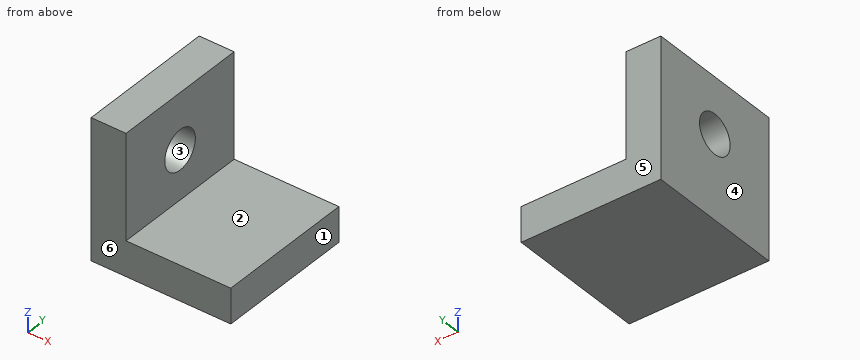
Autodesk Fusion 360 part; units mm, degrees
sketch "Sketch1" plane through (0, 0, 0) normal (0, 0, 1) x (1, 0, 0)
  line L0 (0, 0) -> (25.4, 0)
  line L1 (25.4, 0) -> (25.4, 25.4)
  line L2 (25.4, 25.4) -> (0, 25.4)
  line L3 (0, 25.4) -> (0, 0)
  line L4 (0, 25.4) -> (6.35, 25.4)
  line L5 (6.35, 25.4) -> (6.35, 0)
  line L6 (6.35, 0) -> (0, 0)
  line L7 (0, 0) -> (0, 25.4)
  dimension "d1" = 25.4
  dimension "d2" = 25.4
  dimension "d3" = 6.35
extrude "Extrude1" add sketch "Sketch1" along normal blind 6.35 contours L0 L1 L2 L5
extrude "Extrude2" add sketch "Sketch1" along normal blind 25.4 contours L0 L2 L3 L4 L5 L6 L7
sketch "Sketch2" plane through (6.35, 0, 0) normal (1, 0, 0) x (0, 1, 0)
  line L0 (0, 6.35) -> (25.4, 6.35)
  line L1 (25.4, 6.35) -> (25.4, 25.4)
  line L2 (25.4, 25.4) -> (0, 25.4)
  line L3 (0, 25.4) -> (0, 6.35)
  circle A0 centre (12.7, 15.24) radius 3.5921
extrude "Extrude3" cut sketch "Sketch2" against normal blind 38.1 contours A0
For this review, take the finished solid that the model builds, in its own axes (mm). Face numbers are marked on the shaded views. A direction names the side the tool comes from. Give positions to 0.01 mm unless a question says otherwise; leave off trailing zeros. Loops run counter-clockwise (first coordinate to the right, second up) from the corner with the lowest first, then second, coordinate; pieces in that order, holes last.
Item 1: Take a section at C-C, the plane y = 10. State the section outline as (x, z) points, and give its area (3 significant figures).
Item 2: Insertion check: pin 1 (6 mm diameter, centred on y = 14, z = 22, fed in from +X); pin 2 (5.5 mm diameter, centred on x = 18.5, y = 7.5, fed in from +Z). Each pin has a flat end and moves straight along its axis. Give the tip position at first contact, or say it passes through.
Item 3: Take a section at B-B, the plane z = 15.24. State the section outline as (x, y) points, and give its area (3 significant figures).
Item 4: For line 1 along Z through (x, y) = (2.75, 12.7); line 2 along Z through (x, y) = (20.75, 13.5), list the stretches that pass through material, from the lowest coordinate up.
Item 5: Take a section at A-A, the plane y = 12.7. State the section outline as (x, z) points, and give its area (3 significant figures).
Item 6: Take a section at D-D, the plane z = 10.75. State the section outline as (x, y) points, and give its area (3 significant figures).
Item 7: Tool access review of the marked faces 1 and 2: name each direction out of +Z, -Z, +X, -X, +Y, -Y from which nothing blocks a thin tool from reaching the whole face with its end or side.
Item 8: Draft analysis for pull direction Y (two halves, no side actions). For the marked faces 3, 4, 5 and 6, state which applies: +Y half, -Y half, draft (parallel to the pull), parting line (faces both ways), or undercut.
Calculated:
1. outline: (0, 0) - (25.4, 0) - (25.4, 6.35) - (6.35, 6.35) - (6.35, 12.87) - (0, 12.87) - close; (0, 17.61) - (6.35, 17.61) - (6.35, 25.4) - (0, 25.4) - close
1. area: 252 mm2
2. pin 1: stops at x = 6.35
2. pin 2: stops at z = 6.35
3. outline: (0, 0) - (6.35, 0) - (6.35, 9.11) - (0, 9.11) - close; (0, 16.29) - (6.35, 16.29) - (6.35, 25.4) - (0, 25.4) - close
3. area: 116 mm2
4. line 1: z = 0 to 11.65, 18.83 to 25.4
4. line 2: z = 0 to 6.35
5. outline: (0, 0) - (25.4, 0) - (25.4, 6.35) - (6.35, 6.35) - (6.35, 11.65) - (0, 11.65) - close; (0, 18.83) - (6.35, 18.83) - (6.35, 25.4) - (0, 25.4) - close
5. area: 237 mm2
6. outline: (0, 0) - (6.35, 0) - (6.35, 25.4) - (0, 25.4) - close
6. area: 161 mm2
7. face 1: +Z, -Z, +X, +Y, -Y
7. face 2: +Z, +X, +Y, -Y
8. face 3: undercut
8. face 4: draft
8. face 5: +Y half
8. face 6: -Y half
